The drawing under review shows one solid part. Ordinate dimensions are in mm from its lowest x, y, z. A direction names the side the tool comes from. Give positions to 0.01 mm unless a question says otherwise; leave off trailing zeros. Order: outer loops, then holes, each group sorted by start corner. A loop starts at its lowest first (then second) coordinate and runs counter-clockwise, first axis right, second up. Notation, with made-up numbers: (-1.75, 30) -> (53.25, 30) arc R14 cw to (53.25, 35) -> close; hole circle Ø7 at (76, 9.25). An arc over 180 degrees is marked (long way). Use a Markdown table: item, result. Add a question column.
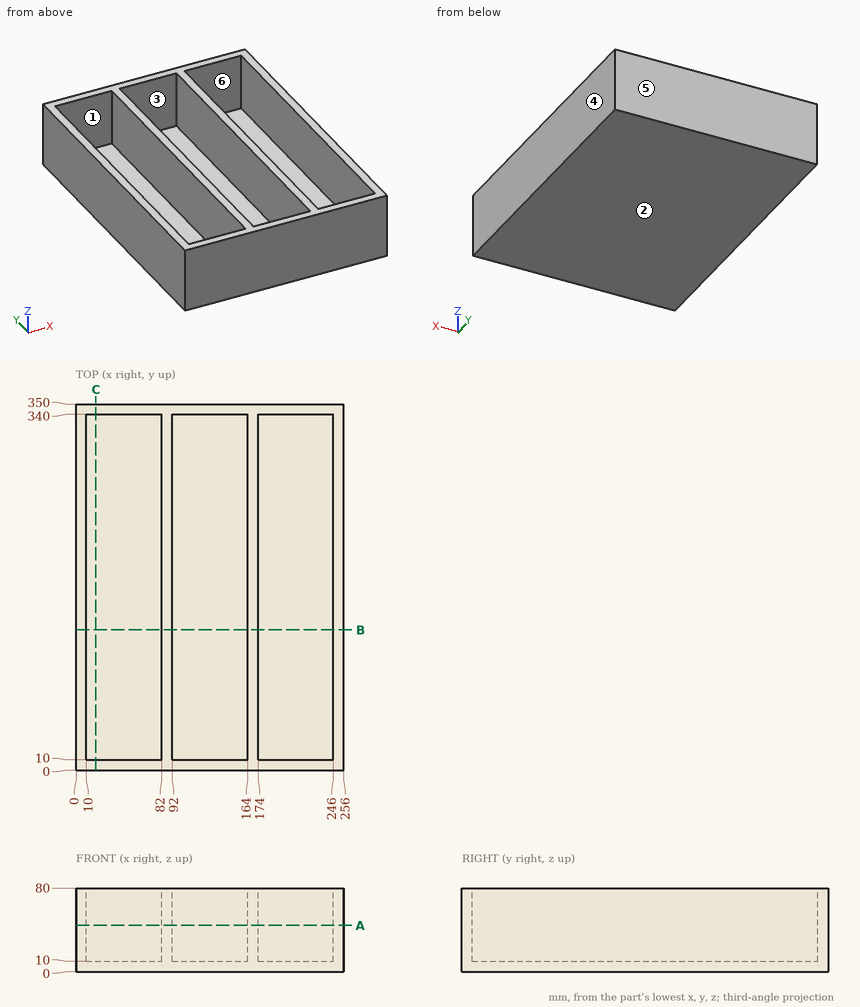
1) Machinability: for the marked faces 1 and 2, which of the approach directions +Z, -Z, +X, -X, +Y, -Y give a long, thin tool a straight path to every point of the face, cutting with its end or side? Answer none if there is none.
2) Insertion check: pin 1 (6 mm diameter, centred on x = 115, z = 37, fed in from -Y); pin 2 (4 mm diameter, centred on x = 157.5, y = 205, fed in from +Z). Each pin has a flat end and moves straight along its axis. Give the tip position at first contact, or say it passes through.
3) The part is to be moulded in two halves that separate along X. For the marked faces 3, 4, 5 and 6, say which applies: +X half, -X half, draft (parallel to the pull), parting line (faces both ways), or undercut.
4) For L1, parallel to X at y = 113, z = 56; L2, parallel to Y at x = 69, z = 45; L3, parallel to Z at x = 79.5, y = 80, list the stretches that pass through material, from the lowest coordinate up. Write a range as [from, to].
5) Add section B-B (y = 134). Give the boundary of the cut face in (x, z).
6) Add section A-A (z = 44.5). Give the boundary of the cut face in (x, y).
7) Add section C-C (x = 19). Give the boundary of the cut face in (y, z).
Worked answers:
| question | item | result |
|---|---|---|
| 1 | face 1 | +Z |
| 1 | face 2 | -Z, +X, -X, +Y, -Y |
| 2 | pin 1 | y = 0 |
| 2 | pin 2 | z = 10 |
| 3 | face 3 | undercut |
| 3 | face 4 | +X half |
| 3 | face 5 | draft |
| 3 | face 6 | undercut |
| 4 | L1 | [0, 10], [82, 92], [164, 174], [246, 256] |
| 4 | L2 | [0, 10], [340, 350] |
| 4 | L3 | [0, 10] |
| 5 | outline | (0, 0) -> (256, 0) -> (256, 80) -> (246, 80) -> (246, 10) -> (174, 10) -> (174, 80) -> (164, 80) -> (164, 10) -> (92, 10) -> (92, 80) -> (82, 80) -> (82, 10) -> (10, 10) -> (10, 80) -> (0, 80) -> close |
| 6 | outline | (0, 0) -> (256, 0) -> (256, 350) -> (0, 350) -> close; hole (10, 10) -> (82, 10) -> (82, 340) -> (10, 340) -> close; hole (92, 10) -> (164, 10) -> (164, 340) -> (92, 340) -> close; hole (174, 10) -> (246, 10) -> (246, 340) -> (174, 340) -> close |
| 7 | outline | (0, 0) -> (350, 0) -> (350, 80) -> (340, 80) -> (340, 10) -> (10, 10) -> (10, 80) -> (0, 80) -> close |
